Can you work these out from the model? Positions are in its coordinate system, mm. A direction names the side the tool comes from. Coordinates: 2 decimals unless noted, no trailing zeros. Order: outer loops, then holes, each group sorted by start corner. A loop starts at its lowest first (then second) coordinate and runs counter-clockwise, first axis right, second up. Notation, with made-up numbers: M 19.5,28 L 37.5,28 A22 cw 37.5,52 Z; hole C 53.25,-25.75 d5. An arc over 180 degrees is marked long. Answer as a JSON object with one key per item and string values.
Autodesk Inventor part; units mm, degrees
ref_plane "YZ Plane" through (0, 0, 0) normal (1, 0, 0) x (0, 1, 0)
ref_plane "XZ Plane" through (0, 0, 0) normal (0, 1, 0) x (-1, 0, 0)
ref_plane "XY Plane" through (0, 0, 0) normal (0, 0, 1) x (1, 0, 0)
sketch "Sketch1" plane through (0, 0, 0) normal (0, 1, 0) x (-1, 0, 0)
  line L0 (0, 0) -> (0, -230)
  line L1 (0, -230) -> (40, -230)
  line L2 (40, -230) -> (40, 0)
  line L3 (40, 0) -> (0, 0)
  dimension "d0" = 230
  dimension "d1" = 40
extrude "Extrusion1" add sketch "Sketch1" along normal blind 5.5
sketch "Sketch2" plane through (0, 5.5, 0) normal (0, 1, 0) x (1, 0, 0)
  line L0 (-40, 0) -> (0, 0) construction
  line L1 (-20, 0) -> (-20, 30) construction
  line L2 (-20, 30) -> (-22.75, 30)
  line L3 (-40, 230) -> (-40, 0) construction
  line L4 (-22.75, 30) -> (-22.75, 80)
  line L5 (-22.75, 80) -> (-20, 80)
  line L6 (-20, 30) -> (-17.25, 30)
  line L7 (-17.25, 30) -> (-17.25, 80)
  line L8 (-17.25, 80) -> (-20, 80)
  dimension "d4" = 30
  dimension "d5" = 2.75
  dimension "d6" = 50
extrude "Extrusion2" cut sketch "Sketch2" against normal blind 5.5
sketch "Sketch3" plane through (0, 5.5, 0) normal (0, 1, 0) x (1, 0, 0)
  line L0 (-40, 0) -> (0, 0) construction
  line L1 (-20, 0) -> (-20, 15) construction
  dimension "d9" = 15
hole "Hole1" at (-20, 5.5, -15) direction (0, -1, 0) diameter 5.9175 depth 19.1 tip angle 118
sketch "Sketch4" plane through (0, 5.5, 0) normal (0, 1, 0) x (1, 0, 0)
  line L0 (0, 230) -> (-40, 230) construction
  line L1 (-20, 230) -> (-20, 140) construction
  point P0 (0, 0)
  dimension "d17" = 90
hole "Hole2" at (-20, 5.5, -140) direction (0, -1, 0) diameter 6.4587 depth 19.1 tip angle 118
properties part number "LMK"
Item 1: I want a section at D-D, the plane z = -15. Write out the boundary of the cut face in (x, y), plus the area to 3 significant figures.
Answers follow:
{"outline": "M -40,0 L -22.96,0 L -22.96,5.5 L -40,5.5 Z; M -17.04,0 L 0,0 L 0,5.5 L -17.04,5.5 Z", "area": "187 mm^2"}
Item 2: I want a section at A-A, the plane z = -39.5. Write out the boundary of the cut face in (x, y), plus the area to 3 significant figures.
Answers follow:
{"outline": "M -40,0 L -22.75,0 L -22.75,5.5 L -40,5.5 Z; M -17.25,0 L 0,0 L 0,5.5 L -17.25,5.5 Z", "area": "190 mm^2"}
Item 3: If we mould it in two halves opening along X, with no side actions, what happens to faces 3 (the flat face through (-20, 0, -113)), 4 (the flat face through (-40, 3, -117)), 5 (the cylindrical face through (-20.89, 2.71, -12.18))? For each: pulls with the +X half, pulls with the -X half, needs draft (parallel to the pull), parting line crosses it, or undercut.
Answers follow:
{"face 3": "needs draft", "face 4": "pulls with the -X half", "face 5": "undercut"}
Item 4: I want a section at B-B, the plane y = 3.4. Write out the boundary of the cut face in (x, z).
Answers follow:
{"outline": "M -40,-230 L 0,-230 L 0,0 L -40,0 Z; hole C -20,-140 d6.46; hole C -20,-15 d5.92; hole M -22.75,-80 L -17.25,-80 L -17.25,-30 L -22.75,-30 Z"}
Item 5: I want a section at C-C, the plane x = -20. Write out the boundary of the cut face in (y, z).
Answers follow:
{"outline": "M 0,-230 L 5.5,-230 L 5.5,-143.23 L 0,-143.23 Z; M 0,-136.77 L 5.5,-136.77 L 5.5,-80 L 0,-80 Z; M 0,-30 L 5.5,-30 L 5.5,-17.96 L 0,-17.96 Z; M 0,-12.04 L 5.5,-12.04 L 5.5,0 L 0,0 Z"}
Item 6: Which directions (+Z, -Z, +X, -X, +Y, -Y) give clear straight access to the entire face, cutting with the end or side of a thin tool? Please do faces 1 (the flat face through (-17.25, 3, -55)), 2 (the flat face through (0, 3, -113)).
Answers follow:
{"face 1": "+Y, -Y", "face 2": "+Z, -Z, +X, +Y, -Y"}
Item 7: Please list where these lines run through material, in increasing order: line 1 (Z direction, x = -20, y = 4.1); line 2 (Z direction, x = -20.5, y = 5); line 3 (X direction, y = 1.3, z = -47).
Answers follow:
{"line 1": "z = -230 to -143.23, -136.77 to -80, -30 to -17.96, -12.04 to 0", "line 2": "z = -230 to -143.19, -136.81 to -80, -30 to -17.92, -12.08 to 0", "line 3": "x = -40 to -22.75, -17.25 to 0"}
